Part print with two shaded views. Sizes in mm from the minimum x, y, z corner. A direction names the side the tool comes from. Round coordinates to 2 decimals unless told otherwise and drop trailing zeros. Order: outer loops, then holes, each group sorted by start corner. A loop starts at its lowest first (then second) coordinate and runs counter-clockwise, first axis right, second up. Notation, with made-up numbers: (0.25, -23) -> (51.25, -23) arc R25 cw to (51.25, 12) -> close; hole circle Ø4 at (-6.5, 62.5). An arc over 180 degrees is marked (long way). Use a Markdown table: item, result. Add a question column.
Item 1: Pin check, flat tips, straight feed: pin 1 (3.5 mm diameter, centred on x = 4, z = 6, fed in from -Y); pin 2 (1.5 mm diameter, centred on x = 1.5, y = 1, fed in from +Z); pin 3 (3 mm diameter, centred on y = 5, z = 1.5, fed in from +X). Stop position of each tip, or through.
Item 2: Two-plate mould, pull along X, no slides. Class the marked faces 1, 2 and 3: released by +X, released by -X, zero draft, split by the parting line, or undercut.
Item 3: 3-axis set-ups, long thin cutter, end or side, ignore diameter. For the marked faces 4 and 5: which of +Z, -Z, +X, -X, +Y, -Y reach the whole face in a straight line?
Item 4: Slice it at A-A, the plane x = 5. Give the cut face in (y, z).
Item 5: Probe L1, parallel to Z at x = 5, y = 1.65; L2, parallel to X at y = 5.05, z = 5. List the from-to ranges inside material, lowest first.
Item 6: Slice it at D-D, the plane y = 3.4. Give the cut face in (x, z).
Item 7: Slice it at C-C, the plane y = 1.75. Give the cut face in (x, z).
Item 8: Slice it at B-B, the plane z = 5. Give the cut face in (x, y), plus the area to 3 significant figures.
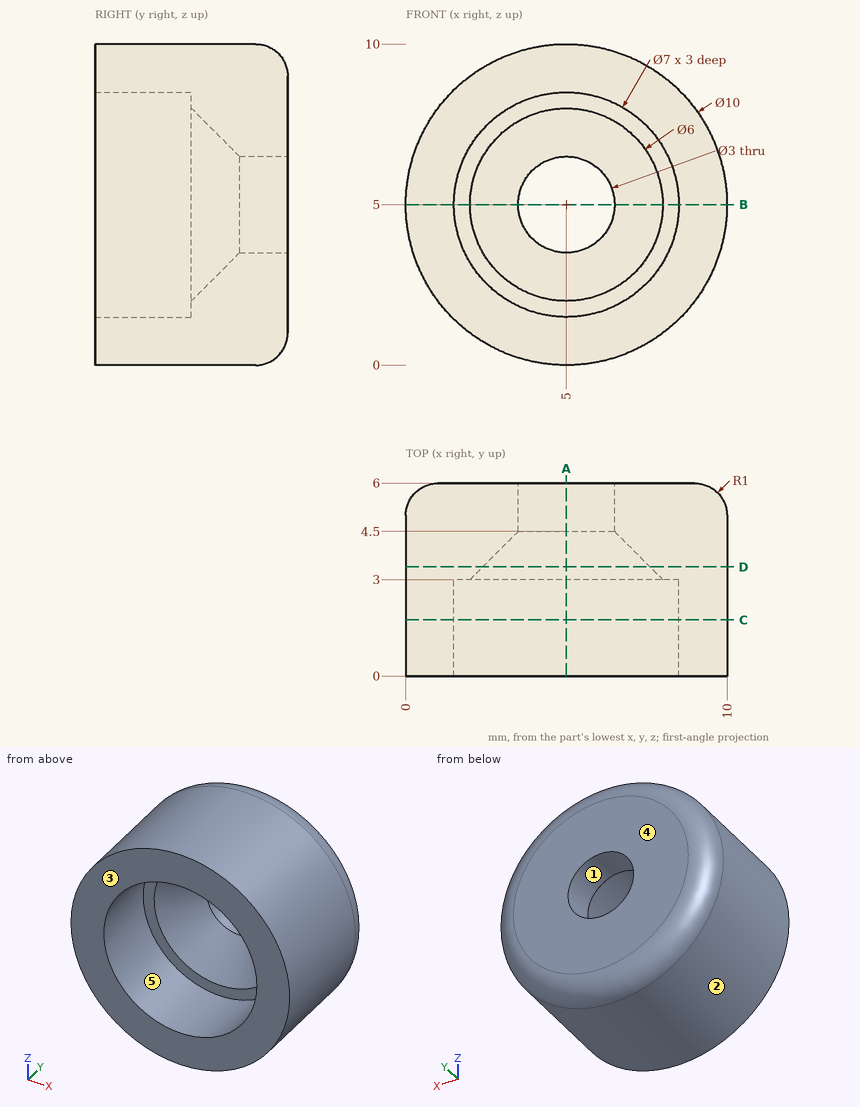
Check sheet entries:
| question | item | result |
|---|---|---|
| 1 | pin 1 | y = 3 |
| 1 | pin 2 | z = 9.18 |
| 1 | pin 3 | x = 9.58 |
| 2 | face 1 | undercut |
| 2 | face 2 | split by the parting line |
| 2 | face 3 | zero draft |
| 3 | face 4 | +Z, -Z, +X, -X, +Y |
| 3 | face 5 | -Y |
| 4 | outline | (0, 0) -> (5, 0) arc R1 ccw to (6, 1) -> (6, 3.5) -> (4.5, 3.5) -> (3, 2) -> (3, 1.5) -> (0, 1.5) -> close; (0, 8.5) -> (3, 8.5) -> (3, 8) -> (4.5, 6.5) -> (6, 6.5) -> (6, 9) arc R1 ccw to (5, 10) -> (0, 10) -> close |
| 5 | L1 | 0 to 1.5, 8.5 to 10 |
| 5 | L2 | 0 to 3.5, 6.5 to 10 |
| 6 | outline | circle Ø10 at (5, 5); hole circle Ø5.2 at (5, 5) |
| 7 | outline | circle Ø10 at (5, 5); hole circle Ø7 at (5, 5) |
| 8 | outline | (0, 0) -> (1.5, 0) -> (1.5, 3) -> (2, 3) -> (3.5, 4.5) -> (3.5, 6) -> (1, 6) arc R1 ccw to (0, 5) -> close; (6.5, 4.5) -> (8, 3) -> (8.5, 3) -> (8.5, 0) -> (10, 0) -> (10, 5) arc R1 ccw to (9, 6) -> (6.5, 6) -> close |
| 8 | area | 27.3 mm2 |
